Verification items for the finished model (mm, model axes). A direction names the side the tool comes from. Coordinates: 2 decimals unless noted, no trailing zeros. Write each loop counter-clockwise with the first axis right and the second up, starting at its lowest first coordinate (ties: lowest second). Pieces come first, ordered by that corner, then holes.
```python
from build123d import *

# Parameters (mm, degrees)
EXTRUDE_1_DEPTH     = 50
SKETCH_2_R          = 1.5
SKETCH_2_R_2        = 1
SKETCH_2_R_3        = 1.05
CUT_EXTRUDE_1_DEPTH = 55.184868737
SKETCH_3_W          = 38
SKETCH_3_H          = 8.212947129
CUT_EXTRUDE_2_DEPTH = 50
FILLET_1_R          = 1


with BuildPart() as part:
    # 草圖1 → 填料-伸長1 (new body)
    with BuildSketch(Plane.XY):
        with BuildLine():
            Line((0, 4), (0, 0))
            Line((0, 0), (20, 0))
            Line((20, 0), (20, -2))
            Line((20, -2), (-12, -2))
            Line((-12, -2), (-12, 4))
            Line((-12, 4), (-5.05, 4))
            ThreePointArc((-5.05, 4), (-3.5, 2.45), (-1.95, 4))
            Line((-1.95, 4), (0, 4))
        make_face()
    extrude(amount=-EXTRUDE_1_DEPTH)

    # 草圖2 → 除料-伸長1 (cut, through all)
    with BuildSketch(Plane(origin=(0, 4, 0), x_dir=(1, 0, 0), z_dir=(0, 1, 0))):
        with Locations(Location((-8.525, 47, 0), (0, 0, 270))):
            Circle(SKETCH_2_R)
        with Locations(Location((-8.525, 3, 0), (0, 0, 270))):
            Circle(SKETCH_2_R)
        with Locations(Location((5.5, 43, 0), (0, 0, 270))):
            Circle(SKETCH_2_R_2)
        with Locations(Location((14.5, 43, 0), (0, 0, 270))):
            Circle(SKETCH_2_R_2)
        with Locations(Location((5.5, 3, 0), (0, 0, 270))):
            Circle(SKETCH_2_R_2)
        with Locations(Location((14.5, 3, 0), (0, 0, 270))):
            Circle(SKETCH_2_R_2)
        with Locations(Location((10, 5.5, 0), (0, 0, 270))):
            Circle(SKETCH_2_R_3)
        with Locations(Location((10, 40.5, 0), (0, 0, 270))):
            Circle(SKETCH_2_R_3)
    extrude(amount=-CUT_EXTRUDE_1_DEPTH, mode=Mode.SUBTRACT)

    # 草圖3 → 除料-伸長2 (cut)
    with BuildSketch(Plane(origin=(0, 0, 0), x_dir=(0, 0, -1), z_dir=(1, 0, 0))):
        with Locations((25, 4.106473564)):
            Rectangle(SKETCH_3_W, SKETCH_3_H)
    extrude(amount=-CUT_EXTRUDE_2_DEPTH, mode=Mode.SUBTRACT)

    # 圓角1
    fillet_1_edges = [part.edges().sort_by_distance(p)[0] for p in [
        (-12, 1, 0),
        (20, -1, -50),
        (0, 2, -50),
        (-12, 1, -50),
        (0, 2, -44),
        (0, 2, -6),
        (0, 2, 0),
        (20, -1, 0),
    ]]
    fillet(fillet_1_edges, radius=FILLET_1_R)


solid = part.part
```
1. Sectioned sample at D-D, the plane y = 1.8. Record the boundary of the cut face in (x, z) (3 decimals), and give its area (3 significant figures).
2. Sectioned sample at A-A, the plane z = -3. Record the boundary of the cut face in (x, y) (3 decimals).
3. Gauge pin test, flat ends, axial feed: P1, Ø3.5, axis at x = 10, z = -5.5, coming from the +Y side; P2, Ø3, axis at y = 2, z = -2, coming from the +X side. Record the tip position at first contact, or that the pin passes through.
4. Sectioned sample at C-C, the plane x = 14.5. Record the boundary of the cut face in (y, z).
5. Material ranges on L1, parallel to X at y = -1.5, z = -43; L2, parallel to X at y = -1, z = -40.5; L3, parallel to Y at x = 15.5, z = -28.5, recorded low to high.
6. Tool access check on faces 1 (the cylindrical face through (-0.285, 1.972, -49.699)), 2 (the cylindrical face through (6.49, -0.99, -3.13)), 3 (the cylindrical face through (-0.285, 1.972, -0.301)), 4 (the flat face through (0, 2, -3)), 5 (the flat face through (4, 0, -25)). Record the directions out of +Z, -Z, +X, -X, +Y, -Y that give a thin tool (end or side, any length) a straight path to the whole face; none if there is none.
7. Draft check along Z on faces 6 (the flat face through (0.9, -0.3, 0)), 7 (the flat face through (-6, 2, -6)), 8 (the flat face through (0.9, -0.3, -50)). Enter one of: pulls with the +Z half, pulls with the -Z half, needs draft (parallel to the pull), parting line crosses it, or undercut.
8. Sectioned sample at B-B, the plane z = -43. Record the boundary of the cut face in (x, y), and give its area (3 significant figures).
Outcome:
1. outline: (-12, -49) arc R1 ccw to (-11, -50) - (-1, -50) arc R1 ccw to (0, -49) - (0, -45) arc R1 ccw to (-1, -44) - (-12, -44) - close; (-12, -6) - (-1, -6) arc R1 ccw to (0, -5) - (0, -1) arc R1 ccw to (-1, 0) - (-11, 0) arc R1 ccw to (-12, -1) - close; hole circle Ø3 at (-8.525, -47); hole circle Ø3 at (-8.525, -3)
1. area: 129 mm2
2. outline: (-12, -2) - (-10.025, -2) - (-10.025, 4) - (-12, 4) - close; (-7.025, -2) - (4.5, -2) - (4.5, 0) - (0, 0) - (0, 4) - (-1.95, 4) arc R1.55 cw to (-5.05, 4) - (-7.025, 4) - close; (6.5, -2) - (13.5, -2) - (13.5, 0) - (6.5, 0) - close; (15.5, -2) - (20, -2) - (20, 0) - (15.5, 0) - close
3. P1: stops at y = 0
3. P2: stops at x = 0
4. outline: (-2, -50) - (0, -50) - (0, -44) - (-2, -44) - close; (-2, -42) - (0, -42) - (0, -4) - (-2, -4) - close; (-2, -2) - (0, -2) - (0, 0) - (-2, 0) - close
5. L1: x = -12 to 4.5, 6.5 to 13.5, 15.5 to 20
5. L2: x = -12 to 8.95, 11.05 to 20
5. L3: y = -2 to 0
6. face 1: -Z, +X, +Y
6. face 2: +Y, -Y
6. face 3: +Z, +X, +Y
6. face 4: +Z, -Z, +X, +Y
6. face 5: +X, +Y
7. face 6: pulls with the +Z half
7. face 7: undercut
7. face 8: pulls with the -Z half
8. outline: (-12, -2) - (4.5, -2) - (4.5, 0) - (-12, 0) - close; (6.5, -2) - (13.5, -2) - (13.5, 0) - (6.5, 0) - close; (15.5, -2) - (20, -2) - (20, 0) - (15.5, 0) - close
8. area: 56.0 mm2
